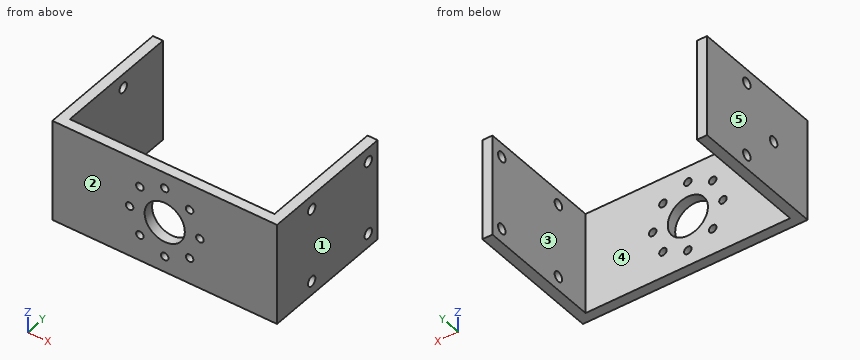
from build123d import *

# Parameters (mm, degrees)
SKETCH1_W               = 44.73
SKETCH1_H               = 20.3
YAWMOUNT_DEPTH          = 2
SKETCH2_W               = 2
SKETCH2_H               = 20.3
BODYCONNECTORS_DEPTH    = 25
SKETCH3_R               = 4
AXLE_COUNTERBORE_DEPTH  = 2
SKETCH5_R               = 0.75
AZEL_MOUNTSCREWS_DEPTH  = 2
SKETCH6_R               = 1
GEARSIDE_SCREWS_DEPTH   = 2
SKETCH7_R               = 1
SMOOTHSIDE_SCREWS_DEPTH = 2


with BuildPart() as part:
    # Sketch1 → YawMount (new body)
    with BuildSketch(Plane(origin=(0, 0, 0), x_dir=(1, 0, 0), z_dir=(0, 1, 0))):
        with Locations((22.365, 10.15)):
            Rectangle(SKETCH1_W, SKETCH1_H)
    extrude(amount=YAWMOUNT_DEPTH)

    # Sketch2 → BodyConnectors (add)
    with BuildSketch(Plane(origin=(0, 2, 0), x_dir=(1, 0, 0), z_dir=(0, 1, 0))):
        with Locations((1, 10.15)):
            Rectangle(SKETCH2_W, SKETCH2_H)
        with Locations((43.73, 10.15)):
            Rectangle(SKETCH2_W, SKETCH2_H)
    extrude(amount=BODYCONNECTORS_DEPTH)

    # Sketch3 → Axle-Counterbore (cut)
    with BuildSketch(Plane.XZ):
        with Locations(Location((22.365, -10.15, 0), (0, 0, 270))):
            Circle(SKETCH3_R)
    extrude(amount=-AXLE_COUNTERBORE_DEPTH, mode=Mode.SUBTRACT)

    # Sketch5 → azel-mountscrews (cut)
    with BuildSketch(Plane.XZ):
        with Locations(Location((15.365, -10.15, 0), (0, 0, 270))):
            Circle(SKETCH5_R)
        with Locations(Location((17.415252532, -5.200252532, 0), (0, 0, 270))):
            Circle(SKETCH5_R)
        with Locations(Location((22.365, -3.15, 0), (0, 0, 270))):
            Circle(SKETCH5_R)
        with Locations(Location((27.314747468, -5.200252532, 0), (0, 0, 270))):
            Circle(SKETCH5_R)
        with Locations(Location((29.365, -10.15, 0), (0, 0, 270))):
            Circle(SKETCH5_R)
        with Locations(Location((27.314747468, -15.099747468, 0), (0, 0, 270))):
            Circle(SKETCH5_R)
        with Locations(Location((22.365, -17.15, 0), (0, 0, 270))):
            Circle(SKETCH5_R)
        with Locations(Location((17.415252532, -15.099747468, 0), (0, 0, 270))):
            Circle(SKETCH5_R)
    extrude(amount=-AZEL_MOUNTSCREWS_DEPTH, mode=Mode.SUBTRACT)

    # Sketch6 → GearSide-Screws (cut)
    with BuildSketch(Plane(origin=(2, 0, 0), x_dir=(0, 0, -1), z_dir=(1, 0, 0))):
        with Locations((10.15, 9.12)):
            Circle(SKETCH6_R)
        with Locations((17.525, 16.33)):
            Circle(SKETCH6_R)
        with Locations((2.775, 16.33)):
            Circle(SKETCH6_R)
    extrude(amount=-GEARSIDE_SCREWS_DEPTH, mode=Mode.SUBTRACT)

    # Sketch7 → SmoothSide-Screws (cut)
    with BuildSketch(Plane.ZY.offset(-42.73)):
        with Locations((-2.775, 9.3)):
            Circle(SKETCH7_R)
        with Locations((-17.525, 9.3)):
            Circle(SKETCH7_R)
        with Locations((-17.525, 24.5)):
            Circle(SKETCH7_R)
        with Locations((-2.775, 24.5)):
            Circle(SKETCH7_R)
    extrude(amount=-SMOOTHSIDE_SCREWS_DEPTH, mode=Mode.SUBTRACT)


solid = part.part
The listing builds one solid part. Answer for the finished solid, in the listing's coordinates (mm). Face numbers are marked on the shaded views. A direction names the side the tool comes from. Coordinates: 2 decimals unless noted, no trailing zeros. Order: outer loops, then holes, each group sorted by start corner. A loop starts at its lowest first (then second) coordinate and runs counter-clockwise, first axis right, second up. Notation, with made-up numbers: (45, 3.25) -> (74, 3.25) arc R20 ccw to (74, 18.25) -> close; hole circle Ø5 at (-26.5, 84). An arc over 180 degrees is marked (long way). Answer in a Markdown table with one row per item. Add a question column.
Item 1: Find section D-D (z = -7). Write down the section's boundary in (x, y), then the cut area to 3 significant figures.
Item 2: Find section A-A (y = 21.5). Write down the section's boundary in (x, z), then the cut area to 3 significant figures.
Item 3: Which of the six approach directions +Z, -Z, +X, -X, +Y, -Y give full straight-line access (tool end or side, diameter ignored) to the marked faces 4 and 5?
Item 4: Find section B-B (z = -17.15). Write down the section's boundary in (x, y) (3 decimals).
Item 5: Each of these flat-tipped pins is pushed along its axis until it touches: P1, Ø1.2, axis at y = 24.5, z = -17.525, coming from the +X side; P2, Ø1.4, axis at x = 17.42, z = -5.2, coming from the +Y side; P3, Ø2.5, axis at x = 22.365, z = -17.15, coming from the -Y side; P4, Ø9, axis at x = 22.365, z = -10.15, coming from the +Y side. Where does it stop, or does it pass through?
Item 6: Find section C-C (y = 16.33). Write down the section's boundary in (x, z) (3 decimals).
Item 7: Determine the mould class of the marked faces 1, 2 and 3 for opening direction X: +X half, -X half, draft (parallel to the pull), parting line (faces both ways), or undercut.
Item 8: Find the intervals of material crossed by L1, parallel to X at y = 0.9, z = -10.15 (3 decimals); L2, parallel to X at y = 10.5, z = -2.25; L3, parallel to Y at x = 1.5, z = -10.15, in increasing order. Write a range as from..to.
Result set:
| question | item | result |
|---|---|---|
| 1 | outline | (0, 0) -> (19.9, 0) -> (19.9, 2) -> (2, 2) -> (2, 27) -> (0, 27) -> close; (24.83, 0) -> (44.73, 0) -> (44.73, 27) -> (42.73, 27) -> (42.73, 2) -> (24.83, 2) -> close |
| 1 | area | 180 mm² |
| 2 | outline | (0, -20.3) -> (2, -20.3) -> (2, 0) -> (0, 0) -> close; (42.73, -20.3) -> (44.73, -20.3) -> (44.73, 0) -> (42.73, 0) -> close |
| 2 | area | 81.2 mm² |
| 3 | face 4 | +Z, -Z, +Y |
| 3 | face 5 | +Z, -Z, -X, +Y, -Y |
| 4 | outline | (0, 0) -> (21.615, 0) -> (21.615, 2) -> (2, 2) -> (2, 15.403) -> (0, 15.403) -> close; (0, 17.257) -> (2, 17.257) -> (2, 27) -> (0, 27) -> close; (23.115, 0) -> (44.73, 0) -> (44.73, 8.373) -> (42.73, 8.373) -> (42.73, 2) -> (23.115, 2) -> close; (42.73, 10.227) -> (44.73, 10.227) -> (44.73, 23.573) -> (42.73, 23.573) -> close; (42.73, 25.427) -> (44.73, 25.427) -> (44.73, 27) -> (42.73, 27) -> close |
| 5 | P1 | stops at x = 2 |
| 5 | P2 | passes through |
| 5 | P3 | stops at y = 0 |
| 5 | P4 | stops at y = 2 |
| 6 | outline | (0, -20.3) -> (2, -20.3) -> (2, -18.525) -> (0, -18.525) -> close; (0, -16.525) -> (2, -16.525) -> (2, -3.775) -> (0, -3.775) -> close; (0, -1.775) -> (2, -1.775) -> (2, 0) -> (0, 0) -> close; (42.73, -20.3) -> (44.73, -20.3) -> (44.73, 0) -> (42.73, 0) -> close |
| 7 | face 1 | +X half |
| 7 | face 2 | draft |
| 7 | face 3 | undercut |
| 8 | L1 | x = 0..14.615, 16.115..18.365, 26.365..28.615, 30.115..44.73 |
| 8 | L2 | x = 0..2, 42.73..44.73 |
| 8 | L3 | y = 0..8.12, 10.12..27 |
